Build history of the part. All positions in model axes, mm. A direction names the side the tool comes from. Round coordinates to 2 decimals unless told otherwise and drop trailing zeros. Loops run counter-clockwise (first coordinate to the right, second up) from the corner with the lowest first, then second, coordinate; pieces in that order, holes last. Notation, with made-up numbers: (-32, 87.5) -> (19, 87.5) arc R24 cw to (19, 110.5) -> close; hole circle Ø2 at (-1, 34). An arc over 180 degrees is marked (long way). Put each result on its own line as item: value. Start each with the question number.
Item 1: Tool access for faces 1 (the flat face through (47, -8, -11)), 2 (the flat face through (38, 7.757, -11)), 3 (the flat face through (-36, 5.4, -22)), 4 (the flat face through (-30.6, -9, -5)): list every direction of +Z, -Z, +X, -X, +Y, -Y with a clear straight run to the whole face (end or side of a thin tool).
Item 2: Cut at B-B, the plane y = 11. List the corners of the cut face in (x, z).
Item 3: Drill centre lines: probe 1 along X at (y, z) = (5.5, -7); probe 2 along Y at (x, z) = (-38.1, -23.3); probe 3 along X at (y, z) = (4.5, -5.25). Where is each one in solid material? Low to high. Write a range as [from, to].
Item 4: Cut at A-A, the plane z = -6.75. List the corners of the cut face in (x, y), plus the area to 3 significant figures.
Item 5: Flat gauge pins, fed straight in: pin 1 Ø8 at (x, y) = (-11.5, -4.5) entering from +Z; pin 2 Ø12 at (x, z) = (42.5, -17) entering from -Y; pin 3 Ø1 at (x, y) = (-47, -9) entering from -Z; pin 4 Ø7.5 at (x, y) = (-39, -0.5) entering from +Z. Where does each tip first touch, or does it go through?
Item 6: Pull direction X, two halves, no side cores. Call faces 5 (the flat face through (0, 0, -22)), 6 (the flat face through (0, -4, -24)), 7 (the flat face through (38, -6.987, -24)): +X half, -X half, draft (parallel to the pull), parting line (faces both ways), or undercut.
Item 7: Cut at D-D, the plane z = -20.5. List the corners of the cut face in (x, y).
Item 8: Cut at C-C, the plane x = 14. List the corners of the cut face in (y, z).
```python
from build123d import *

# Parameters (mm, degrees)
F0_R      = 13
F2_DEPTH  = 26
F3_DEPTH  = 22
F5_DEPTH  = 30
F7_W      = 53
F7_H      = 8
F8_DEPTH  = 4
F9_W      = 25
F9_H      = 5
F10_DEPTH = 15


with BuildPart() as f2:
    # F0 (on Top) → F2 (new body)
    with BuildSketch(Plane.XY):
        with Locations((-38.1, 0)):
            Circle(F0_R)
    extrude(amount=-F2_DEPTH)


with BuildPart() as f2b:
    # F0 (on Top) → F2, piece 2 (new body)
    with BuildSketch(Plane.XY):
        with BuildLine():
            ThreePointArc((51.1, 0), (38.1, 13), (25.1, 0))
            ThreePointArc((25.1, 0), (38.1, -13), (51.1, 0))
        make_face()
    extrude(amount=-F2_DEPTH)


with BuildPart() as f3_tool:
    # F1 (on Top) → F3 (new body)
    with BuildSketch(Plane.XY):
        with BuildLine():
            ThreePointArc((-31.4, -7.7570935279), (-28.779659341, -4.2654132273), (-27.85, 0))
            Line((-27.85, 0), (-31.4, 0))
            Line((-31.4, 0), (-31.4, -7.7570935279))
        make_face()
        with BuildLine():
            Line((-31.4, 0), (-27.85, 0))
            ThreePointArc((-27.85, 0), (-28.779659341, 4.2654132273), (-31.4, 7.7570935279))
            Line((-31.4, 7.7570935279), (-31.4, 0))
        make_face()
        Polygon((-31.4, -7.7570935279), (-31.4, 0), (-31.4, 7.7570935279), (-44.8, 7.7570935279), (-44.8, -7.7570935279), align=None)
        with BuildLine():
            Line((-44.8, -7.7570935279), (-44.8, 7.7570935279))
            ThreePointArc((-44.8, 7.7570935279), (-48.35, 0), (-44.8, -7.7570935279))
        make_face()
        Polygon((31.4, 7.7570935279), (31.4, 0), (31.4, -7.7570935279), (44.8, -7.7570935279), (44.8, 7.7570935279), align=None)
        with BuildLine():
            ThreePointArc((48.35, 0), (47.420340659, 4.2654132273), (44.8, 7.7570935279))
            Line((44.8, 7.7570935279), (44.8, -7.7570935279))
            ThreePointArc((44.8, -7.7570935279), (47.420340659, -4.2654132273), (48.35, 0))
        make_face()
        with BuildLine():
            Line((31.4, -7.7570935279), (31.4, 0))
            Line((31.4, 0), (27.85, 0))
            ThreePointArc((27.85, 0), (28.779659341, -4.2654132273), (31.4, -7.7570935279))
        make_face()
        with BuildLine():
            Line((27.85, 0), (31.4, 0))
            Line((31.4, 0), (31.4, 7.7570935279))
            ThreePointArc((31.4, 7.7570935279), (28.779659341, 4.2654132273), (27.85, 0))
        make_face()
    extrude(amount=-F3_DEPTH)


with BuildPart() as f2_1:
    add(f2.part)

    # F3: cut by f3_tool
    add(f3_tool.part, mode=Mode.SUBTRACT)


with BuildPart() as f2b_1:
    add(f2b.part)

    # F3: cut by f3_tool
    add(f3_tool.part, mode=Mode.SUBTRACT)


with BuildPart() as f5_tool:
    # F4 (on Top) → F5 (new body)
    with BuildSketch(Plane.XY):
        with BuildLine():
            ThreePointArc((-38.1, -5.5), (-34.2109127035, -3.8890872965), (-32.6, 0))
            Line((-32.6, 0), (-38.1, 0))
            Line((-38.1, 0), (-38.1, -5.5))
        make_face()
        Polygon((45.6, -6.9865943062), (38.1, -6.9865943062), (30.6, -6.9865943062), (30.6, -13), (45.6, -13), align=None)
        with BuildLine():
            ThreePointArc((43.6, 0), (38.1, 5.5), (32.6, 0))
            Line((32.6, 0), (38.1, 0))
            Line((38.1, 0), (38.1, -5.5))
            ThreePointArc((38.1, -5.5), (41.9890872965, -3.8890872965), (43.6, 0))
        make_face()
        with BuildLine():
            Line((38.1, 0), (32.6, 0))
            ThreePointArc((32.6, 0), (34.2109127035, -3.8890872965), (38.1, -5.5))
            Line((38.1, -5.5), (38.1, 0))
        make_face()
        with BuildLine():
            Line((-38.1, 0), (-32.6, 0))
            ThreePointArc((-32.6, 0), (-41.9890872965, 3.8890872965), (-38.1, -5.5))
            Line((-38.1, -5.5), (-38.1, 0))
        make_face()
        Polygon((-30.6, -6.9865943062), (-38.1, -6.9865943062), (-45.6, -6.9865943062), (-45.6, -13), (-30.6, -13), align=None)
    extrude(amount=-F5_DEPTH)


with BuildPart() as f2_2:
    add(f2_1.part)

    # F5: cut by f5_tool
    add(f5_tool.part, mode=Mode.SUBTRACT)



with BuildPart() as f2b_2:
    add(f2b_1.part)

    # F5: cut by f5_tool
    add(f5_tool.part, mode=Mode.SUBTRACT)


with BuildPart() as f2_3:
    add(f2_2.part)

    add(f2b_2.part)  # F8 merges F2b
    # F7 (on offset) → F8 (join)
    with BuildSketch(Plane.XY.offset(-26)):
        Rectangle(F7_W, F7_H)
    extrude(amount=F8_DEPTH)

    # F9 (on offset) → F10 (cut)
    with BuildSketch(Plane.XY.offset(-26)):
        with Locations((-38.1, -9.4865943062)):
            Rectangle(F9_W, F9_H)
        with Locations((38.1, -9.4865943062)):
            Rectangle(F9_W, F9_H)
    extrude(amount=F10_DEPTH, mode=Mode.SUBTRACT)


solid = f2_3.part
```
Reply:
1. face 1: -Z, +X, -X, -Y
1. face 2: +Z, -Y
1. face 3: +Z
1. face 4: +Z, -Z, -Y
2. outline: (-45.03, -26) -> (-31.17, -26) -> (-31.17, 0) -> (-45.03, 0) -> close; (31.17, -26) -> (45.03, -26) -> (45.03, 0) -> (31.17, 0) -> close
3. probe 1: x = [-49.88, -46.75], [-29.45, -26.32], [26.32, 29.45], [46.75, 49.88]
3. probe 2: y = [-6.99, -5.5], [5.5, 13]
3. probe 3: x = [-50.3, -47.31], [-28.89, -25.9], [25.9, 28.89], [47.31, 50.3]
4. outline: (-45.6, -10.62) -> (-45.6, -6.99) arc R10.25 cw to (-44.8, 7.76) -> (-31.4, 7.76) arc R10.25 cw to (-30.6, -6.99) -> (-30.6, -10.62) arc R13 ccw (long way) to start; (30.6, -10.62) -> (30.6, -6.99) arc R10.25 cw to (31.4, 7.76) -> (44.8, 7.76) arc R10.25 cw to (45.6, -6.99) -> (45.6, -10.62) arc R13 ccw (long way) to start
4. area: 358 mm^2
5. pin 1: stops at z = -22
5. pin 2: stops at y = -6.99
5. pin 3: stops at z = -11
5. pin 4: passes through
6. face 5: undercut
6. face 6: undercut
6. face 7: draft
7. outline: (-49.06, -6.99) -> (-45.6, -6.99) arc R10.25 cw to (-44.8, 7.76) -> (-31.4, 7.76) arc R10.25 cw to (-30.6, -6.99) -> (-27.14, -6.99) arc R13 ccw (long way) to start; (27.14, -6.99) -> (30.6, -6.99) arc R10.25 cw to (31.4, 7.76) -> (44.8, 7.76) arc R10.25 cw to (45.6, -6.99) -> (49.06, -6.99) arc R13 ccw (long way) to start
8. outline: (-4, -26) -> (4, -26) -> (4, -22) -> (-4, -22) -> close
